Read the model definition and answer for the solid it produces. Units are mm, in the model's axes. A direction names the side the tool comes from. Give positions to 0.01 mm unless a question says otherwise; leave off trailing zeros. Order: outer loops, then holes, each group sorted by start corner. A loop starts at its lowest first (then second) coordinate and runs counter-clockwise, first axis right, second up.
Autodesk Fusion 360 part; units mm, degrees
sketch "Sketch1" plane through (0, 0, 0) normal (0, 1, 0) x (1, 0, 0)
  line L0 (-50.8, 25.4) -> (50.8, 25.4)
  line L1 (50.8, 25.4) -> (50.8, -25.4)
  line L2 (50.8, -25.4) -> (-50.8, -25.4)
  line L3 (-50.8, -25.4) -> (-50.8, 25.4)
  line L4 (-50.8, -25.4) -> (50.8, 25.4)
  line L5 (-50.8, 25.4) -> (50.8, -25.4)
  dimension "d1" = 50.8
  dimension "d2" = 101.6
extrude "Extrude1" add sketch "Sketch1" along normal blind 9.5
sketch "Sketch2" plane through (0, 9.5, 0) normal (0, 1, 0) x (-1, 0, 0)
  line L0 (50.8, 25.4) -> (-50.8, 25.4)
  line L1 (-50.8, 25.4) -> (-50.8, -25.4)
  line L2 (-50.8, -25.4) -> (50.8, -25.4)
  line L3 (50.8, -25.4) -> (50.8, 25.4)
  line L4 (50.8, -2.5) -> (-50.8, -2.5)
  line L5 (-50.8, -2.5) -> (-50.8, 2.5)
  line L6 (-50.8, 2.5) -> (50.8, 2.5)
  line L7 (50.8, 2.5) -> (50.8, -2.5)
  line L8 (50.8, 2.5) -> (-50.8, -2.5)
  dimension "d5" = 5
extrude "Extrude2" add sketch "Sketch2" along normal blind 38.1 contours L1 L5 L6 L8 | L3 L4 L7 L8
sketch "Sketch3" plane through (0, 9.5, 0) normal (0, 1, 0) x (-1, 0, 0)
  line L0 (-50.8, 2.5) -> (50.8, 2.5)
  line L1 (50.8, 2.5) -> (50.8, 25.4)
  line L2 (50.8, 25.4) -> (-50.8, 25.4)
  line L3 (-50.8, 25.4) -> (-50.8, 2.5)
  line L4 (41.3, 10.575) -> (-41.3, 10.575)
  line L5 (-41.3, 10.575) -> (-41.3, 17.325)
  line L6 (-41.3, 17.325) -> (41.3, 17.325)
  line L7 (41.3, 17.325) -> (41.3, 10.575)
  line L8 (0, 2.5) -> (0, 10.575)
  line L9 (0, 17.325) -> (0, 25.4)
  line L10 (41.3, 13.95) -> (50.8, 13.95)
  line L11 (-41.3, 13.95) -> (-50.8, 13.95)
  line L12 (41.341, -18.4703) -> (-41.259, -18.4703)
  line L13 (-41.259, -18.4703) -> (-41.259, -11.7203)
  line L14 (-41.259, -11.7203) -> (41.341, -11.7203)
  line L15 (41.341, -11.7203) -> (41.341, -18.4703)
  line L16 (0.041, -26.5453) -> (0.041, -18.4703)
  dimension "d8" = 82.6
  dimension "d9" = 6.75
extrude "Extrude3" cut sketch "Sketch3" against normal blind 20 contours L4 L5 L6 L7 | L12 L13 L14 L15
hole "Hole1" at (-41.3, 9.5, 13.95) direction (0, -1, 0) diameter 6.75 depth 30 tip angle 118
hole "Hole2" at (-41.341, 9.5, -15.0953) direction (0, -1, 0) diameter 6.75 depth 30 tip angle 118
hole "Hole3" at (41.259, 9.5, -15.0953) direction (0, -1, 0) diameter 6.75 depth 30 tip angle 118
hole "Hole4" at (41.3, 9.5, 13.95) direction (0, -1, 0) diameter 6.75 depth 30 tip angle 118
sketch "Sketch4" plane through (0, 0, 0) normal (0, -1, 0) x (1, 0, 0)
  arc A0 (41.259, -18.4703) -> (41.259, -11.7203) centre (41.259, -15.0953) ccw
  line L0 (41.259, -18.4703) -> (-41.341, -18.4703)
  arc A1 (-41.341, -11.7203) -> (-41.341, -18.4703) centre (-41.341, -15.0953) ccw
  line L1 (-41.341, -11.7203) -> (41.259, -11.7203)
  arc A2 (41.3, 10.575) -> (41.3, 17.325) centre (41.3, 13.95) ccw
  line L2 (41.3, 10.575) -> (-41.3, 10.575)
  arc A3 (-41.3, 17.325) -> (-41.3, 10.575) centre (-41.3, 13.95) ccw
  line L3 (-41.3, 17.325) -> (41.3, 17.325)
  line L4 (50.8, 25.4) -> (-50.8, 25.4)
  line L5 (-50.8, 25.4) -> (-50.8, -25.4)
  line L6 (-50.8, -25.4) -> (50.8, -25.4)
  line L7 (50.8, -25.4) -> (50.8, 25.4)
  line L8 (-50.8, 7) -> (50.8, 7)
  line L9 (50.8, 7) -> (50.8, -7)
  line L10 (50.8, -7) -> (-50.8, -7)
  line L11 (-50.8, -7) -> (-50.8, 7)
  line L12 (-50.8, 0) -> (50.8, 0)
  line L13 (0, 7) -> (0, -7)
  dimension "d25" = 101.6
  dimension "d26" = 14
extrude "Extrude4" cut sketch "Sketch4" against normal blind 2 contours L7 L8 L9 L12 L13 | L5 L8 L11 L12 L13 | L7 L9 L10 L12 L13 | L5 L10 L11 L12 L13
sketch "Sketch5" plane through (0, 0, -2.5) normal (0, 0, -1) x (-1, 0, 0)
  line L0 (-50.8, 9.5) -> (50.8, 9.5)
  line L1 (50.8, 9.5) -> (50.8, 47.6)
  line L2 (50.8, 47.6) -> (-50.8, 47.6)
  line L3 (-50.8, 47.6) -> (-50.8, 9.5)
  circle A0 centre (-38.1, 32.142) radius 4.85
  circle A1 centre (-12.7, 32.142) radius 4.8997
  circle A2 centre (12.7, 32.142) radius 4.85
  circle A3 centre (38.1, 32.142) radius 4.85
  line L4 (-38.1, 32.142) -> (-12.7, 32.142)
  line L5 (-12.7, 32.142) -> (12.7, 32.142)
  line L6 (12.7, 32.142) -> (38.1, 32.142)
  line L7 (-42.95, 37.0417) -> (42.95, 37.0417)
  line L8 (42.95, 37.0417) -> (42.95, 28.1917)
  line L9 (42.95, 28.1917) -> (-42.95, 28.1917)
  line L10 (-42.95, 28.1917) -> (-42.95, 37.0417)
  line L11 (42.95, 32.6167) -> (50.8, 32.6167)
  line L12 (-42.95, 32.6167) -> (-50.8, 32.6167)
  dimension "d29" = 9.7
  dimension "d31" = 8.85
  dimension "d32" = 25.4
extrude "Extrude5" cut sketch "Sketch5" against normal blind 20 contours A0 L9 | A3 L9 | A1 L4 L5 | A1 L4 L5 L9 | A2 L5 L6 | A2 L5 L6 L9 picked at (-39.4169, 32.3517) picked at (37.6141, 31.8651)
equation "d8 = 101.6 mm - 19 mm"
1) The part is cut by section B-B on z = 13.95. Determine the outline of the cut face in (x, y) (3 decimals).
Final values:
outline: (-50.8, 0) - (-44.675, 0) - (-44.675, 9.5) - (-50.8, 9.5) - close; (44.675, 0) - (50.8, 0) - (50.8, 9.5) - (44.675, 9.5) - close
2) Given pin 1 (11.5 mm diameter, centred on x = 12.7, y = 32.142, fed in from +Z); pin 2 (8 mm diameter, centred on x = -29.5, y = 35.5, fed in from -Z); pin 3 (4 mm diameter, centred on x = 10.5, z = 1.5, fed in from -Y), each flat-ended and moving along its own axis, determine where each tip first touches the part or whether it passes through.
Final values:
pin 1: stops at z = 2.5
pin 2: stops at z = -2.5
pin 3: stops at y = 2
3) Consider L1, parallel to Z at x = -23, y = 8 (3 decimals); L2, parallel to Y at x = 12, z = 1; L3, parallel to Z at x = -21, y = 22. Determine where each line is inside the solid, lowest interval first.
Final values:
L1: z = -25.4 to -18.47, -11.72 to 10.575, 17.325 to 25.4
L2: y = 2 to 28.19, 36.99 to 47.6
L3: z = -2.5 to 2.5
4) The part is cut by section A-A on x = 5.5. Determine the outline of the cut face in (y, z) (3 decimals), and give its area (3 significant figures).
Final values:
outline: (0, -25.4) - (9.5, -25.4) - (9.5, -18.47) - (0, -18.47) - close; (0, -11.72) - (9.5, -11.72) - (9.5, -2.5) - (47.6, -2.5) - (47.6, 2.5) - (9.5, 2.5) - (9.5, 10.575) - (0, 10.575) - (0, 7) - (2, 7) - (2, -7) - (0, -7) - close; (0, 17.325) - (9.5, 17.325) - (9.5, 25.4) - (0, 25.4) - close
area: 517 mm2
5) The part is cut by section D-D on y = 31. Determine the outline of the cut face in (x, z), and give its area (3 significant figures).
Final values:
outline: (-50.8, -2.5) - (-42.81, -2.5) - (-42.81, 2.5) - (-50.8, 2.5) - close; (-33.39, -2.5) - (-17.41, -2.5) - (-17.41, 2.5) - (-33.39, 2.5) - close; (-7.99, -2.5) - (7.94, -2.5) - (7.94, 2.5) - (-7.99, 2.5) - close; (17.46, -2.5) - (33.39, -2.5) - (33.39, 2.5) - (17.46, 2.5) - close; (42.81, -2.5) - (50.8, -2.5) - (50.8, 2.5) - (42.81, 2.5) - close
area: 319 mm2
6) The part is cut by section C-C on x = 38.1. Determine the outline of the cut face in (y, z) (3 decimals), and give its area (3 significant figures).
Final values:
outline: (0, -25.4) - (9.5, -25.4) - (9.5, -18.47) - (0, -18.47) - close; (0, -11.72) - (9.5, -11.72) - (9.5, -2.5) - (28.192, -2.5) - (28.192, 2.5) - (9.5, 2.5) - (9.5, 10.575) - (0, 10.575) - (0, 7) - (2, 7) - (2, -7) - (0, -7) - close; (0, 17.325) - (9.5, 17.325) - (9.5, 25.4) - (0, 25.4) - close; (36.992, -2.5) - (47.6, -2.5) - (47.6, 2.5) - (36.992, 2.5) - close
area: 473 mm2
7) For a pull along X with two mould halves and no side action, classify faces 4 (the face through (50.8, 11, 0)), 5 (the face through (38, 28.192, 0)), 6 (the face through (1, 28, 2.5)) as released by +X, released by -X, zero draft, split by the parting line, or undercut.
Final values:
face 4: released by +X
face 5: undercut
face 6: zero draft
8) A tool of negligible diameter and unlimited length cuts with its end or side. For faces 1 (the face through (-1, 2, 0)), 2 (the face through (-1, 28, -2.5)), 3 (the face through (1, 5, -11.72)), from which of +Z, -Z, +X, -X, +Y, -Y can it reach the whole face along a straight path? Write none if from no direction.
Final values:
face 1: +X, -X, -Y
face 2: -Z, +X, -X, +Y
face 3: +Y, -Y
